from build123d import *

# Parameters (mm, degrees)
F1_DEPTH       = 5
F5_D           = 4.5
F5_CBORE_D     = 8.25
F5_CBORE_DEPTH = 3.5


with BuildPart() as f1:
    # F0 (on Top) → F1 (new body, symmetric)
    with BuildSketch(Plane.XY):
        with BuildLine():
            ThreePointArc((7.8784620241, 9.8445622258), (5.5480407874, 5.6168738236), (7.8784620241, 1.3891854213))
            ThreePointArc((7.8784620241, 1.3891854213), (6.128355545, -5.1423008775), (0, -8))
            Line((0, -8), (0, -11))
            ThreePointArc((0, -11), (8.2547271195, -7.2704525432), (10.9119275962, 1.3891854213))
            ThreePointArc((10.9119275962, 1.3891854213), (13.2423488329, 5.6168738236), (10.9119275962, 9.8445622258))
            ThreePointArc((10.9119275962, 9.8445622258), (9.3951948102, 11.3803842849), (7.8784620241, 9.8445622258))
        make_face()
        with BuildLine():
            Line((-4.8236730193, -8), (0, -8))
            ThreePointArc((0, -8), (-6.128355545, -5.1423008775), (-7.8784620241, 1.3891854213))
            ThreePointArc((-7.8784620241, 1.3891854213), (-5.5480407874, 5.6168738236), (-7.8784620241, 9.8445622258))
            ThreePointArc((-7.8784620241, 9.8445622258), (-9.3951948102, 11.3803842849), (-10.9119275962, 9.8445622258))
            ThreePointArc((-10.9119275962, 9.8445622258), (-13.2423488329, 5.6168738236), (-10.9119275962, 1.3891854213))
            ThreePointArc((-10.9119275962, 1.3891854213), (-10.0626974149, -4.4432106339), (-6.3245553203, -9))
            Line((-6.3245553203, -9), (-5, -9))
            Line((-5, -9), (-4.8236730193, -8))
        make_face()
        with BuildLine():
            Line((0, -11), (0, -8))
            Line((0, -8), (-4.8236730193, -8))
            Line((-4.8236730193, -8), (-5, -9))
            Line((-5, -9), (-6.3245553203, -9))
            ThreePointArc((-6.3245553203, -9), (-3.3166247904, -10.4880884817), (0, -11))
        make_face()
    extrude(amount=F1_DEPTH, both=True)


with BuildPart() as f2:
    # F0 (on Top) → F2 (revolve)
    with BuildSketch(Plane.XY):
        with BuildLine():
            Line((0, -11), (0, -8))
            Line((0, -8), (-4.8236730193, -8))
            Line((-4.8236730193, -8), (-5, -9))
            Line((-5, -9), (-6.3245553203, -9))
            ThreePointArc((-6.3245553203, -9), (-3.3166247904, -10.4880884817), (0, -11))
        make_face()
        with BuildLine():
            Line((0, -14), (0, -11))
            ThreePointArc((0, -11), (-3.3166247904, -10.4880884817), (-6.3245553203, -9))
            Line((-6.3245553203, -9), (-15, -9))
            Line((-15, -9), (-15, -14))
            Line((-15, -14), (0, -14))
        make_face()
    revolve(axis=Axis((0, -31.6533013247, 0), (0, -1, 0)))


with BuildPart() as f1_1:
    add(f1.part)

    # F3: union F2
    add(f2.part)

    # F5 (through all)
    with Locations(Plane(origin=(0, -9, 0), x_dir=(-1, 0, 0), z_dir=(0, 1, 0))):
        with Locations((0, -10), (0, 10)):
            CounterBoreHole(F5_D / 2, F5_CBORE_D / 2, F5_CBORE_DEPTH)


solid = f1_1.part
CAD build for the part. Positions are in the model's coordinates, mm. A direction names the side the tool comes from. Coordinates: 2 decimals unless noted, no trailing zeros. Loops run counter-clockwise (first coordinate to the right, second up) from the corner with the lowest first, then second, coordinate; pieces in that order, holes last. Notation, with made-up numbers: (30, 26.5) - (50, 26.5) arc R15 cw to (50, 31.5) - close; hole circle Ø10 at (65.5, -0.75). An arc over 180 degrees is marked (long way). Use one line per item in the form item = value. Start each with the question number.
1) Band-saw the part on A-A (y = 0). Give the cut face in (x, z).
2) Band-saw the part on C-C (z = -10). Give the cut face in (x, y) (3 decimals), and give its area (3 significant figures).
3) Band-saw the part on B-B (x = -12.25). Give the cut face in (y, z).
4) Flat gauge pins, fed straight in: pin 1 (14.5 mm diameter, centred on x = 0, y = 0, fed in from +Z); pin 2 (1 mm diameter, centred on x = 10, y = -9.5, fed in from -Z); pin 3 (2 mm diameter, centred on x = 7, y = -9, fed in from -Z); pin 4 (3.5 mm diameter, centred on x = 0, z = 10, fed in from +Y). Where does each tip first touch, or does it go through?
5) Drill centre lines: L1, parallel to Z at x = 0, y = -11.3 (3 decimals); L2, parallel to X at y = 0, z = -1; L3, parallel to Y at x = -9.5, z = 2.5. Where is each one in solid material? Low to high. Write a range as from..to.
6) Tool access for faces 4 (the face through (-6, 4, 5)), 5 (the face through (-2, -12.5, 8)), 6 (the face through (-6, 4, -5)): list every direction of +Z, -Z, +X, -X, +Y, -Y with a clear straight run to the whole face (end or side of a thin tool).
7) Band-saw the part on D-D (z = 0). Give the cut face in (x, y), and give its area (3 significant figures).
8) Two-plate mould, pull along X, no slides. Class faces 1 (the face through (13.24, 5.55, 0.07)), 2 (the face through (5.55, 5.69, 0.07)), 3 (the face through (0, -14, 0)): +X half, -X half, draft (parallel to the pull), parting line (faces both ways), or undercut.
Check values:
q1.outline = (-11, -5) - (-8, -5) - (-8, 5) - (-11, 5) - close; (8, -5) - (11, -5) - (11, 5) - (8, 5) - close
q2.outline = (-11.18, -14) - (-2.25, -14) - (-2.25, -12.5) - (-4.125, -12.5) - (-4.125, -9) - (-11.18, -9) - close; (2.25, -14) - (11.18, -14) - (11.18, -9) - (4.125, -9) - (4.125, -12.5) - (2.25, -12.5) - close
q2.area = 76.2 mm2
q3.outline = (-14, -8.66) - (-9, -8.66) - (-9, 8.66) - (-14, 8.66) - close; (2.63, -5) - (8.61, -5) - (8.61, 5) - (2.63, 5) - close
q4.pin_1 = 5
q4.pin_2 = -11.61
q4.pin_3 = -13.75
q4.pin_4 = through
q5.L1 = -15..-14.125, -5.875..5.875, 14.125..15
q5.L2 = -11..-8, 8..11
q5.L3 = -14..-9, -5.55..11.38
q6.face_4 = +Z, +X, -X, +Y
q6.face_5 = +Y
q6.face_6 = -Z, +X, -X, +Y
q7.outline = (-15, -14) - (15, -14) - (15, -9) - (6.32, -9) arc R11 ccw to (10.91, 1.39) arc R5 ccw to (10.91, 9.84) arc R1.52 ccw (long way) to (7.88, 9.84) arc R5 ccw to (7.88, 1.39) arc R8 cw (long way) to (-7.88, 1.39) arc R5 ccw to (-7.88, 9.84) arc R1.52 ccw (long way) to (-10.91, 9.84) arc R5 ccw to (-10.91, 1.39) arc R11 ccw to (-6.32, -9) - (-15, -9) - close
q7.area = 345 mm2
q8.face_1 = +X half
q8.face_2 = undercut
q8.face_3 = draft
